Geometry: final body of the model. Coordinates: model frame, mm. Round coordinates to 2 decimals unless told otherwise and drop trailing zeros. Write each loop counter-clockwise with the first axis right and the second up, starting at its lowest first coordinate (ties: lowest second). Pieces come first, ordered by that corner, then holes. Notation, with made-up numbers: (59.5, 45) - (93.5, 45) arc R9 cw to (93.5, 57) - close; hole circle Ø9 at (-33, -10). An arc over 180 degrees is marked (long way). Write each question's results on one line, items separated by ' | '.
from build123d import *

# Parameters (mm, degrees)
BOSS_EXTRUDE1_DEPTH = 3.175
FILLET1_R           = 3.175
FILLET2_R           = 12.7


with BuildPart() as part:
    # Sketch1 → Boss-Extrude1 (new body)
    with BuildSketch(Plane(origin=(48.385492731365964, 0, 0), x_dir=(0, 0, -1), z_dir=(1, 0, 0))):
        with BuildLine():
            Line((-147.36118847527575, 146.91537779675497), (-111.88055506155092, 203.68439125871458))
            Line((-111.88055506155092, 203.68439125871458), (105.39733503272873, 203.68439125871458))
            Line((105.39733503272873, 203.68439125871458), (140.8779684464535, 146.91537779675497))
            ThreePointArc((140.8779684464535, 146.91537779675497), (123.3774034475485, 150.95396971957916), (119.33881152472429, 133.45340472067417))
            Line((119.33881152472429, 133.45340472067417), (91.31944493844902, 178.28439125871458))
            Line((91.31944493844902, 178.28439125871458), (-97.80266496727123, 178.28439125871458))
            Line((-97.80266496727123, 178.28439125871458), (-125.82203155354657, 133.45340472067417))
            ThreePointArc((-125.82203155354657, 133.45340472067417), (-129.8606234763708, 150.95396971957913), (-147.36118847527575, 146.91537779675497))
        make_face()
    extrude(amount=BOSS_EXTRUDE1_DEPTH)

    # Fillet1
    fillet1_edges = [part.edges().sort_by_distance(p)[0] for p in [
        (49.97299273136596, 146.91537779675497, 147.36118847527575),
        (49.97299273136596, 146.91537779675497, -140.8779684464535),
        (49.97299273136596, 133.45340472067417, -119.33881152472429),
        (49.97299273136596, 133.45340472067417, 125.82203155354657),
    ]]
    fillet(fillet1_edges, radius=FILLET1_R)

    # Fillet2
    fillet2_edges = [part.edges().sort_by_distance(p)[0] for p in [
        (49.97299273136596, 203.68439125871458, 111.88055506155092),
        (49.97299273136596, 203.68439125871458, -105.39733503272873),
        (49.97299273136596, 178.28439125871458, -91.31944493844902),
        (49.97299273136596, 178.28439125871458, 97.80266496727123),
    ]]
    fillet(fillet2_edges, radius=FILLET2_R)


solid = part.part
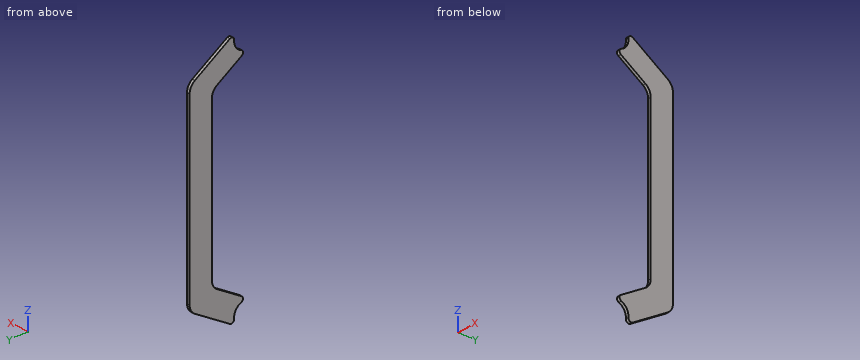
Q1. Section query B-B, the plane z = -41. Return loops of the section in (x, y), plus the area to 3 significant figures.
Answer block:
outline: (48.39, 178.28) - (51.56, 178.28) - (51.56, 203.68) - (48.39, 203.68) - close | area: 80.6 mm2
Q2. Pin query (flat end, axial travel): pin 1 (1 mm diameter, centred on x = 50, z = 15, fed in from -Y). Return the tip coordinate at first contact, or that it passes through.
Answer block:
pin 1: y = 178.28
Q3. Section query C-C, the plane y = 184.5. Return loops of the section in (x, z), plus the area to 3 significant figures.
Answer block:
outline: (48.39, -117.39) - (51.56, -117.39) - (51.56, 123.87) - (48.39, 123.87) - close | area: 766 mm2
Q4. Section query A-A, the plane y = 163. Return loops of the section in (x, z), plus the area to 3 significant figures.
Answer block:
outline: (48.39, -130.83) - (51.56, -130.83) - (51.56, -100.87) - (48.39, -100.87) - close; (48.39, 107.36) - (51.56, 107.36) - (51.56, 137.31) - (48.39, 137.31) - close | area: 190 mm2
Q5. Ray query, line 1 along Y through (x, z) = (50.15, -16); line 2 along Z through (x, y) = (49, 165); line 3 along Z through (x, y) = (49.7, 173.5). Return the intervals inside material, ascending.
Answer block:
line 1: 178.28 to 203.68 | line 2: -129.58 to -99.62, 106.11 to 136.06 | line 3: -124.26 to -94.21, 100.7 to 130.75
